Could you check a few things on this model? Use its own coordinates, in mm. Face numbers are marked on the shaded views. Coordinates: 2 decimals unless noted, no trailing zeros. Write each loop counter-clockwise with the first axis right and the second up, starting at its lowest first coordinate (ties: lowest second). Pieces come first, ordered by that corner, then holes.
Autodesk Inventor part; units mm, degrees
ref_plane "YZ Plane" through (0, 0, 0) normal (1, 0, 0) x (0, 1, 0)
ref_plane "XZ Plane" through (0, 0, 0) normal (0, 1, 0) x (-1, 0, 0)
ref_plane "XY Plane" through (0, 0, 0) normal (0, 0, 1) x (1, 0, 0)
sketch "スケッチ1" plane through (0, 0, 0) normal (0, 0, 1) x (1, 0, 0)
  arc A0 (-17.9, -5.9192) -> (-17.6, -6.2192) centre (-17.6, -5.9192) ccw construction
  line L0 (-17.6, -6.2192) -> (-11.8244, -6.2192) construction
  line L1 (-11.8244, -6.2192) -> (-9.5, -2.219)
  arc A1 (-9.2172, -2.0192) -> (-9.5, -2.219) centre (-9.2172, -2.3192) ccw
  line L2 (-9.2172, -2.0192) -> (-6.9328, -2.0192)
  arc A2 (-6.65, -2.219) -> (-6.9328, -2.0192) centre (-6.9328, -2.3192) ccw
  line L3 (-6.65, -2.219) -> (-4.3256, -6.2192)
  line L4 (-4.3256, -6.2192) -> (8.4756, -6.2192) construction
  line L5 (8.4756, -6.2192) -> (10.8, -2.219)
  arc A3 (11.0828, -2.0192) -> (10.8, -2.219) centre (11.0828, -2.3192) ccw
  line L6 (11.0828, -2.0192) -> (13.3672, -2.0192)
  arc A4 (13.65, -2.219) -> (13.3672, -2.0192) centre (13.3672, -2.3192) ccw
  line L7 (13.65, -2.219) -> (15.9744, -6.2192)
  line L8 (15.9744, -6.2192) -> (21.25, -6.2192) construction
  arc A5 (21.25, -6.2192) -> (21.55, -5.9192) centre (21.25, -5.9192) ccw construction
  line L9 (21.55, -2.3692) -> (21.55, -5.9192) construction
  arc A6 (21.55, -2.3692) -> (21.25, -2.0692) centre (21.25, -2.3692) ccw construction
  line L10 (21.25, -2.0692) -> (17.65, -2.0692) construction
  arc A7 (17.65, 2.2308) -> (17.65, -2.0692) centre (17.65, 0.0808) ccw construction
  line L11 (17.65, 2.2308) -> (21.25, 2.2308) construction
  arc A8 (21.25, 2.2308) -> (21.55, 2.5308) centre (21.25, 2.5308) ccw construction
  line L12 (21.55, 4.8808) -> (21.55, 2.5308) construction
  line L13 (21.55, 4.8808) -> (-17.9, 4.8808) construction
  line L14 (-17.9, 4.8808) -> (-17.9, -5.9192) construction
  line L15 (1.3, 1.9308) -> (1.3, -1.7692) construction
  arc A9 (1, -2.0692) -> (1.3, -1.7692) centre (1, -1.7692) ccw construction
  line L16 (1, -2.0692) -> (-2.5, -2.0692) construction
  arc A10 (-2.5, 2.2308) -> (-2.5, -2.0692) centre (-2.5, 0.0808) ccw construction
  line L17 (-2.5, 2.2308) -> (1, 2.2308) construction
  arc A11 (1.3, 1.9308) -> (1, 2.2308) centre (1, 1.9308) ccw construction
  line L18 (-17.9, 5.3808) -> (21.55, 5.3808) construction
  circle A12 centre (-0.85, 0.0808) radius 2.15 construction
  line L19 (-0.85, 0.0808) -> (-2.5, 0.0808) construction
  circle A13 centre (-1.675, 0.0808) radius 2.25
  line L20 (64.025, 2.5048) -> (64.025, 91.3712) construction
  line L21 (-65.975, 91.3712) -> (-65.975, 2.5048) construction
  line L22 (64.025, 5.3808) -> (-65.975, 5.3808)
  circle A14 centre (18.625, 0.0808) radius 2.25
  circle A15 centre (38.925, 0.0808) radius 2.25
  circle A16 centre (59.225, 0.0808) radius 2.25
  circle A17 centre (-21.975, 0.0808) radius 2.25
  circle A18 centre (-1.675, 0.0808) radius 2.25
  circle A19 centre (18.625, 0.0808) radius 2.25
  circle A20 centre (38.925, 0.0808) radius 2.25
  circle A21 centre (-42.275, 0.0808) radius 2.25
  circle A22 centre (-21.975, 0.0808) radius 2.25
  circle A23 centre (-1.675, 0.0808) radius 2.25
  circle A24 centre (18.625, 0.0808) radius 2.25
  circle A25 centre (-62.575, 0.0808) radius 2.25
  circle A26 centre (-42.275, 0.0808) radius 2.25
  circle A27 centre (-21.975, 0.0808) radius 2.25
  circle A28 centre (-1.675, 0.0808) radius 2.25
  line L23 (64.025, 5.3808) -> (64.025, -6.2192)
  line L24 (64.025, -6.2192) -> (-65.975, -6.2192)
  line L25 (-65.975, -6.2192) -> (-65.975, 5.3808)
  point P0 (0, 0)
  dimension "d1" = 4.5
  dimension "d4" = 20.3
  dimension "d7" = 20.3
extrude "押し出し1" add sketch "スケッチ1" along normal blind 5 contours L24 L25 L22 L23 L7 A4 L6 A3 L5 L3 A2 L2 A1 L1 | L1 A1 L2 A2 L3 L24 | L5 A3 L6 A4 L7 L24 | A16 | A25
sketch "スケッチ3" plane through (0, 0, 0) normal (0, 0, -1) x (-1, 0, 0)
  line L0 (9.5, -2.219) -> (11.8244, -6.2192)
  arc A0 (9.5, -2.219) -> (9.2172, -2.0192) centre (9.2172, -2.3192) ccw
  line L1 (6.9328, -2.0192) -> (9.2172, -2.0192)
  arc A1 (6.9328, -2.0192) -> (6.65, -2.219) centre (6.9328, -2.3192) ccw
  line L2 (4.3256, -6.2192) -> (6.65, -2.219)
  line L3 (65.975, -6.2192) -> (-64.025, -6.2192)
  point P0 (0, 0)
extrude "押し出し2" cut sketch "スケッチ3" against normal through all
pattern_linear "矩形状パターン1" count 4 spacing 20.3 along (1, 0, 0) count 3 spacing 20.3 along (-1, 0, 0) of "押し出し2"
fillet "フィレット1" radius 1 1 edges at (-0.975, 5.3808, 0)
sketch "スケッチ7" plane through (0, 0, 5) normal (0, 0, 1) x (1, 0, 0)
  line L0 (-52.4244, -6.2192) -> (-50.1, -2.219)
  arc A0 (-49.8172, -2.0192) -> (-50.1, -2.219) centre (-49.8172, -2.3192) ccw
  line L1 (-49.8172, -2.0192) -> (-47.5328, -2.0192)
  arc A1 (-47.25, -2.219) -> (-47.5328, -2.0192) centre (-47.5328, -2.3192) ccw
  line L2 (-47.25, -2.219) -> (-44.9256, -6.2192)
  line L3 (-32.1244, -6.2192) -> (-29.8, -2.219)
  arc A2 (-29.5172, -2.0192) -> (-29.8, -2.219) centre (-29.5172, -2.3192) ccw
  line L4 (-29.5172, -2.0192) -> (-27.2328, -2.0192)
  arc A3 (-26.95, -2.219) -> (-27.2328, -2.0192) centre (-27.2328, -2.3192) ccw
  line L5 (-26.95, -2.219) -> (-24.6256, -6.2192)
  line L6 (-11.8244, -6.2192) -> (-9.5, -2.219)
  arc A4 (-9.2172, -2.0192) -> (-9.5, -2.219) centre (-9.2172, -2.3192) ccw
  line L7 (-9.2172, -2.0192) -> (-6.9328, -2.0192)
  arc A5 (-6.65, -2.219) -> (-6.9328, -2.0192) centre (-6.9328, -2.3192) ccw
  line L8 (-6.65, -2.219) -> (-4.3256, -6.2192)
  line L9 (8.4756, -6.2192) -> (10.8, -2.219)
  arc A6 (11.0828, -2.0192) -> (10.8, -2.219) centre (11.0828, -2.3192) ccw
  line L10 (11.0828, -2.0192) -> (13.3672, -2.0192)
  arc A7 (13.65, -2.219) -> (13.3672, -2.0192) centre (13.3672, -2.3192) ccw
  line L11 (13.65, -2.219) -> (15.9744, -6.2192)
  line L12 (28.7756, -6.2192) -> (31.1, -2.219)
  arc A8 (31.3828, -2.0192) -> (31.1, -2.219) centre (31.3828, -2.3192) ccw
  line L13 (31.3828, -2.0192) -> (33.6672, -2.0192)
  arc A9 (33.95, -2.219) -> (33.6672, -2.0192) centre (33.6672, -2.3192) ccw
  line L14 (33.95, -2.219) -> (36.2744, -6.2192)
  line L15 (49.0756, -6.2192) -> (51.4, -2.219)
  arc A10 (51.6828, -2.0192) -> (51.4, -2.219) centre (51.6828, -2.3192) ccw
  line L16 (51.6828, -2.0192) -> (53.9672, -2.0192)
  arc A11 (54.25, -2.219) -> (53.9672, -2.0192) centre (53.9672, -2.3192) ccw
  line L17 (54.25, -2.219) -> (56.5744, -6.2192)
  line L18 (-52.4244, -6.2192) -> (-44.9256, -6.2192)
  line L19 (-24.6256, -6.2192) -> (-26.95, -2.219)
  line L20 (-32.1244, -6.2192) -> (-24.6256, -6.2192)
  line L21 (-9.5, -2.219) -> (-11.8244, -6.2192)
  line L22 (-11.8244, -6.2192) -> (-4.3256, -6.2192)
  line L23 (15.9744, -6.2192) -> (8.4756, -6.2192)
  line L24 (36.2744, -6.2192) -> (33.95, -2.219)
  line L25 (28.7756, -6.2192) -> (36.2744, -6.2192)
  line L26 (49.0756, -6.2192) -> (56.5744, -6.2192)
  point P0 (0, 0)
extrude "押し出し5" add sketch "スケッチ7" against normal blind 4
sketch "スケッチ8" plane through (0, 0, 5) normal (0, 0, 1) x (1, 0, 0)
  circle A0 centre (-42.275, 0.0808) radius 2.25
  circle A1 centre (-21.975, 0.0808) radius 2.25
  line L0 (-42.275, 0.0808) -> (-21.975, 0.0808) construction
  line L1 (-21.975, 0.0808) -> (-32.125, 0.0808) construction
  line L2 (-48.675, -4.6192) -> (-28.375, -4.6192) construction
  circle A2 centre (-48.675, -4.6192) radius 2.25
  circle A3 centre (-28.375, -4.6192) radius 2.25
  line L3 (-65.975, -6.2192) -> (64.025, -6.2192)
  line L4 (-58.675, -6.2192) -> (-18.375, -6.2192)
  line L5 (-18.375, -6.2192) -> (-18.375, -14.6192)
  line L6 (-18.375, -14.6192) -> (-58.675, -14.6192)
  line L7 (-58.675, -14.6192) -> (-58.675, -6.2192)
  line L8 (-65.975, 5.3808) -> (64.025, 5.3808)
  line L9 (-27.2328, -2.0192) -> (-29.5172, -2.0192) construction
  point P0 (0, 0)
  point P1 (-38.525, -14.6192)
  point P2 (-18.375, -6.2192)
  point P3 (-38.525, -4.6192)
  point P4 (-28.375, -2.0192)
  point P5 (-28.375, -2.0192)
  dimension "d43" = 20.3
  dimension "d44" = 4.5
  dimension "d45" = 10
  dimension "d46" = 10
  dimension "d53" = 6.4
  dimension "d54" = 10
  dimension "d62" = 4.5
  dimension "d63" = 20.3
extrude "押し出し6" add sketch "スケッチ8" against normal up to surface (4 mm away) contours A2 L3 A3 L5 L6 L7
sketch "スケッチ10" plane through (0, 0, 5) normal (0, 0, 1) x (1, 0, 0)
  arc A0 (-50.2569, -6.2192) -> (-47.0931, -6.2192) centre (-48.675, -4.6192) ccw construction
  arc A1 (-29.9569, -6.2192) -> (-26.7931, -6.2192) centre (-28.375, -4.6192) ccw construction
  circle A2 centre (-48.675, -4.6192) radius 2.25
  circle A3 centre (-28.375, -4.6192) radius 2.25
  point P0 (0, 0)
extrude "押し出し8" cut sketch "スケッチ10" against normal through all
sketch "スケッチ11" plane through (0, 0, 1) normal (0, 0, -1) x (-1, 0, 0)
  circle A0 centre (28.375, -4.6192) radius 2.25 construction
  circle A1 centre (48.675, -4.6192) radius 2.25 construction
  circle A2 centre (28.375, -4.6192) radius 4.15
  circle A3 centre (48.675, -4.6192) radius 4.15
  point P0 (0, 0)
  dimension "d57" = 8.3
extrude "押し出し9" cut sketch "スケッチ11" along normal blind 10 and the other way blind 1
sketch "スケッチ9" plane through (0, 0, 0) normal (0, 0, -1) x (-1, 0, 0)
  line L0 (58.675, -14.6192) -> (58.675, -6.2192)
  line L1 (58.675, -14.6192) -> (88.3695, -14.6192)
  line L2 (88.3695, -14.6192) -> (88.3695, 31.2927)
  line L3 (88.3695, 31.2927) -> (58.675, 31.2927)
  line L4 (58.675, 31.2927) -> (58.675, -14.6192)
  line L5 (18.375, -14.6192) -> (-64.2943, -14.6192)
  line L6 (-64.2943, -14.6192) -> (-64.2943, 35.8918)
  line L7 (-64.2943, 35.8918) -> (18.375, 35.8918)
  line L8 (18.375, 35.8918) -> (18.375, -14.6192)
  circle A0 centre (21.975, 0.0808) radius 2.25 construction
  line L9 (65.975, 5.3808) -> (-64.025, 5.3808) construction
  circle A1 centre (21.975, 0.0808) radius 5.3 construction
  line L10 (16.675, 5.3808) -> (16.675, -4.5192)
  line L11 (16.675, -4.5192) -> (18.375, -6.2192)
  line L12 (24.5458, -6.2192) -> (11.8244, -6.2192)
  line L13 (16.675, 5.3808) -> (18.375, 5.3808)
  point P0 (0, 0)
  dimension "d64" = 45
extrude "押し出し7" cut sketch "スケッチ9" against normal through all contours L0 L4 L3 L2 L1 | L5 L6 L7 L8 L13 L10 L11
fillet "フィレット2" radius 0.6 5 edges at (-32.2042, -6.2192, 0.5) (-24.5458, -6.2192, 0.5) (-52.5042, -6.2192, 0.5) (-44.8458, -6.2192, 0.5) (-58.675, -6.2192, 0.5)
fillet "フィレット2" radius 1 6 edges at (-58.675, -14.6192, 3) (-18.375, -14.6192, 3) (-58.675, 5.3808, 3) (-16.675, 5.3808, 3) (-16.675, -4.5192, 2.5) (-18.375, -6.2192, 3)
equation "\"d43\" = d63"
properties part number "gpu_hold_plate"
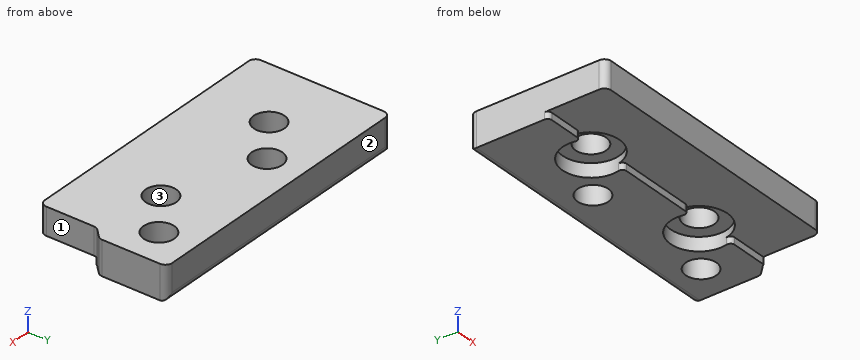
1. For pin 1 (2 mm diameter, centred on x = -41.5, y = -10, fed in from -Z); pin 2 (2.5 mm diameter, centred on x = -29, y = -6.5, fed in from -Z); pin 3 (0.8 mm diameter, centred on x = -19.5, z = 0.5, fed in from -Y); pin 4 (3.5 mm diameter, centred on x = -48.68, y = -4.62, fed in from -Z), each with a flat end and sliding along its axis, tell me the tip position at first contact or that it passes through.
Verdict:
pin 1: stops at z = 1
pin 2: stops at z = 2
pin 3: stops at y = -6.22
pin 4: passes through
2. I want a section at C-C on z = 1.45. Please give me the cut outline in (x, y) (3 decimals), plus the area to 3 significant figures.
Verdict:
outline: (-58.675, -13.619) arc R1 ccw to (-57.675, -14.619) - (-19.375, -14.619) arc R1 ccw to (-18.375, -13.619) - (-18.375, -6.633) arc R1 cw to (-18.082, -5.926) - (-16.968, -4.812) arc R1 ccw to (-16.675, -4.105) - (-16.675, 4.381) arc R1 ccw to (-17.675, 5.381) - (-57.675, 5.381) arc R1 ccw to (-58.675, 4.381) - close; hole circle Ø8.3 at (-48.675, -4.619); hole circle Ø4.5 at (-42.275, 0.081); hole circle Ø8.3 at (-28.375, -4.619); hole circle Ø4.5 at (-21.975, 0.081)
area: 683 mm2
3. I want a section at A-A on y = 1.75. Please give me the cut outline in (x, z) (3 decimals).
Verdict:
outline: (-58.675, 0) - (-43.784, 0) - (-43.784, 5) - (-58.675, 5) - close; (-40.766, 0) - (-23.484, 0) - (-23.484, 5) - (-40.766, 5) - close; (-20.466, 0) - (-16.675, 0) - (-16.675, 5) - (-20.466, 5) - close
4. I want a section at D-D on x = -33.5. Please give me the cut outline in (y, z), plus the area to 3 significant figures.
Verdict:
outline: (-14.62, 1) - (-6.22, 1) - (-6.22, 0) - (4.38, 0) arc R1 ccw to (5.38, 1) - (5.38, 5) - (-14.62, 5) - close
area: 91.4 mm2
5. Please list where these lines run through material, in increasing order: line 1 along X through (y, z) = (-1.25, 2.45) (3 decimals); line 2 along X through (y, z) = (-2.75, 3.05) (3 decimals); line 3 along X through (y, z) = (-1, 0.5) (3 decimals).
Verdict:
line 1: x = -58.675 to -44.089, -40.461 to -23.789, -20.161 to -16.675
line 2: x = -58.675 to -49.927, -47.423 to -29.627, -27.123 to -16.675
line 3: x = -58.675 to -50.706, -46.644 to -44.248, -40.302 to -30.406, -26.344 to -23.948, -20.002 to -16.675
6. I want a section at B-B on x = -50. Please give me the cut outline in (y, z).
Verdict:
outline: (-14.62, 1) - (-8.55, 1) - (-8.55, 2) - (-6.44, 2) - (-6.44, 5) - (-14.62, 5) - close; (-2.8, 2) - (-0.69, 2) - (-0.69, 0) - (4.38, 0) arc R1 ccw to (5.38, 1) - (5.38, 5) - (-2.8, 5) - close
7. If we mould it in two halves opening along X, with no side actions, what happens to the marked faces 1, 2 and 3? For each: pulls with the +X half, pulls with the -X half, needs draft (parallel to the pull), parting line crosses it, or undercut.
Verdict:
face 1: pulls with the +X half
face 2: needs draft
face 3: undercut
